```python
from build123d import *

# Parameters (mm, degrees)
F0_R     = 11.0625
F1_DEPTH = 11
F2_R     = 5
F3_SIZE  = 2
F4_SIZE  = 2


# Not quite as in the source:
# - a feature names something its author has since deleted; it is built from what else it names


with BuildPart() as f1:
    # F0 (on Top) → F1 (new body)
    with BuildSketch(Plane.XY):
        Polygon((12.7279220614, 42.7279220614), (0, 48), (-12.7279220614, 42.7279220614), (-18, 30), (-12.7279220614, 17.2720779386), (-21.3220193017, 2.3866648732), (-34.9807621135, 0.5884572681), (-43.3674269867, -10.3412571882), (-41.5692193817, -24), (-30.6395049254, -32.3866648732), (-16.9807621135, -30.5884572681), (-8.5940972403, -19.6587428118), (8.5940972403, -19.6587428118), (16.9807621135, -30.5884572681), (30.6395049254, -32.3866648732), (41.5692193817, -24), (43.3674269867, -10.3412571882), (34.9807621135, 0.5884572681), (21.3220193017, 2.3866648732), (12.7279220614, 17.2720779386), (18, 30), align=None)
        with Locations((-25.9807621135, -15)):
            Circle(F0_R, mode=Mode.SUBTRACT)
        Circle(F0_R, mode=Mode.SUBTRACT)
        with Locations((25.9807621135, -15)):
            Circle(F0_R, mode=Mode.SUBTRACT)
        with Locations((0, 30)):
            Circle(F0_R, mode=Mode.SUBTRACT)
    extrude(amount=F1_DEPTH)

    # F2
    f2_edges = [f1.edges().sort_by_distance(p)[0] for p in [
        (-16.980762, -30.588457, 5.5),
        (-30.639505, -32.386665, 5.5),
        (-41.569219, -24, 5.5),
        (-43.367427, -10.341257, 5.5),
        (-34.980762, 0.588457, 5.5),
        (-18, 30, 5.5),
        (-12.727922, 42.727922, 5.5),
        (0, 48, 5.5),
        (12.727922, 42.727922, 5.5),
        (34.980762, 0.588457, 5.5),
        (43.367427, -10.341257, 5.5),
        (41.569219, -24, 5.5),
        (30.639505, -32.386665, 5.5),
        (16.980762, -30.588457, 5.5),
        (8.594097, -19.658743, 5.5),
        (-8.594097, -19.658743, 5.5),
        (18, 30, 5.5),
        (-12.727922, 17.272078, 5.5),
        (-21.322019, 2.386665, 5.5),
    ]]
    fillet(f2_edges, radius=F2_R)

    # F3
    f3_edges = [f1.edges().sort_by_distance(p)[0] for p in [
        (27.124716, 1.622725, 11),
        (34.774782, 0.231689, 11),
        (17.024971, 9.829371, 11),
        (39.174095, -4.8764, 11),
        (14.967679, 22.67933, 11),
        (42.969503, -10.447881, 11),
        (17.588039, 30, 11),
        (42.468323, -17.170629, 11),
        (15.363961, 36.363961, 11),
        (41.212451, -23.794019, 11),
        (12.436622, 42.436622, 11),
        (36.104362, -28.193332, 11),
        (6.363961, 45.363961, 11),
        (30.532882, -31.988741, 11),
        (0, 47.588039, 11),
        (23.810134, -31.487561, 11),
        (-6.363961, 45.363961, 11),
        (17.186743, -30.231689, 11),
        (-12.436622, 42.436622, 11),
        (12.907556, -25.280152, 11),
        (-15.363961, 36.363961, 11),
        (8.339814, -20.174379, 11),
        (-17.588039, 30, 11),
        (0, -19.658743, 11),
        (-15.439476, 23.818348, 11),
        (-8.339814, -20.174379, 11),
        (-13.301618, 17.30968, 11),
        (-12.907556, -25.280152, 11),
        (-17.024971, 9.829371, 11),
        (-17.186743, -30.231689, 11),
        (-21.641432, 2.864699, 11),
        (-23.810134, -31.487561, 11),
        (-28.347032, 1.461804, 11),
        (-30.532882, -31.988741, 11),
        (-34.774782, 0.231689, 11),
        (-36.104362, -28.193332, 11),
        (-39.174095, -4.8764, 11),
        (-41.212451, -23.794019, 11),
        (-42.969503, -10.447881, 11),
        (-42.468323, -17.170629, 11),
        (-37.043262, -15, 11),
        (-11.0625, 0, 11),
        (14.918262, -15, 11),
        (-11.0625, 30, 11),
    ]]
    chamfer(f3_edges, length=F3_SIZE)

    # F4
    f4_edges = [f1.edges().sort_by_distance(p)[0] for p in [
        (27.124716, 1.622725, 0),
        (34.774782, 0.231689, 0),
        (17.024971, 9.829371, 0),
        (39.174095, -4.8764, 0),
        (14.967679, 22.67933, 0),
        (42.969503, -10.447881, 0),
        (17.588039, 30, 0),
        (42.468323, -17.170629, 0),
        (15.363961, 36.363961, 0),
        (41.212451, -23.794019, 0),
        (12.436622, 42.436622, 0),
        (36.104362, -28.193332, 0),
        (6.363961, 45.363961, 0),
        (30.532882, -31.988741, 0),
        (0, 47.588039, 0),
        (23.810134, -31.487561, 0),
        (-6.363961, 45.363961, 0),
        (17.186743, -30.231689, 0),
        (-12.436622, 42.436622, 0),
        (12.907556, -25.280152, 0),
        (-15.363961, 36.363961, 0),
        (8.339814, -20.174379, 0),
        (-17.588039, 30, 0),
        (0, -19.658743, 0),
        (-15.439476, 23.818348, 0),
        (-8.339814, -20.174379, 0),
        (-13.301618, 17.30968, 0),
        (-12.907556, -25.280152, 0),
        (-17.024971, 9.829371, 0),
        (-17.186743, -30.231689, 0),
        (-21.641432, 2.864699, 0),
        (-23.810134, -31.487561, 0),
        (-28.347032, 1.461804, 0),
        (-30.532882, -31.988741, 0),
        (-34.774782, 0.231689, 0),
        (-36.104362, -28.193332, 0),
        (-39.174095, -4.8764, 0),
        (-41.212451, -23.794019, 0),
        (-42.969503, -10.447881, 0),
        (-42.468323, -17.170629, 0),
        (-37.043262, -15, 0),
        (-11.0625, 0, 0),
        (14.918262, -15, 0),
        (-11.0625, 30, 0),
    ]]
    chamfer(f4_edges, length=F4_SIZE)


solid = f1.part
```
Verification items for the finished model (mm, model axes). A direction names the side the tool comes from. Round coordinates to 2 decimals unless told otherwise and drop trailing zeros. Order: outer loops, then holes, each group sorted by start corner. A loop starts at its lowest first (then second) coordinate and runs counter-clockwise, first axis right, second up. Notation, with made-up numbers: (82.25, 4.5) - (129.25, 4.5) arc R31 cw to (129.25, 38.5) - close; hole circle Ø6 at (10.25, -31). An arc over 180 degrees is marked (long way). Use CSV: the item, a comma, the result in double quotes.
(1) Thickness scan on probe 1 along Y at (x, z) = (0, 6.5); probe 2 along Y at (x, z) = (4, 3.5); probe 3 along X at (y, z) = (-25, 1.5). Record the ranges inside material, lowest first. Write a range as from..to.
Entries:
probe 1,"-19.66..-11.06, 11.06..18.94, 41.06..47.59"
probe 2,"-19.66..-10.31, 10.31..19.69, 40.31..46.34"
probe 3,"-39.44..-31.79, -20.18..-13.32, 13.32..20.18, 31.79..39.44"
(2) Access from +Z, -Z, +X, -X, +Y, -Y to the whole of each face (thin tool, end or side, straight path). Record for faces 1 (the face through (-24.006, -30.519, 1.014)), 2 (the face through (8.37, -20.19, 5.55)), 3 (the face through (13.65, -24.629, 9.986)), 4 (the face through (16.238, 9.22, 9.986)).
Entries:
face 1,"-Z, -Y"
face 2,"+Z, -Z, -Y"
face 3,"+Z, -Y"
face 4,"+Z, +X"
(3) Section check A-A on x = 0. Record the boundary of the cut face in (y, z).
Entries:
outline,"(-19.66, 2) - (-17.66, 0) - (-13.06, 0) - (-11.06, 2) - (-11.06, 9) - (-13.06, 11) - (-17.66, 11) - (-19.66, 9) - close; (11.06, 2) - (13.06, 0) - (16.94, 0) - (18.94, 2) - (18.94, 9) - (16.94, 11) - (13.06, 11) - (11.06, 9) - close; (41.06, 2) - (43.06, 0) - (45.59, 0) - (47.59, 2) - (47.59, 9) - (45.59, 11) - (43.06, 11) - (41.06, 9) - close"
(4) Section check C-C on y = -15. Record the boundary of the cut face in (x, z).
Entries:
outline,"(-42.75, 2) - (-40.74, 0) - (-39.04, 0) - (-37.04, 2) - (-37.04, 9) - (-39.04, 11) - (-40.74, 11) - (-42.75, 9) - close; (-14.92, 2) - (-12.92, 0) - (12.92, 0) - (14.92, 2) - (14.92, 9) - (12.92, 11) - (-12.92, 11) - (-14.92, 9) - close; (37.04, 2) - (39.04, 0) - (40.74, 0) - (42.75, 2) - (42.75, 9) - (40.74, 11) - (39.04, 11) - (37.04, 9) - close"
(5) Gauge pin test, flat ends, axial feed: pin 1 Ø2 at (y, z) = (-23, 8) entering from -X; pin 2 Ø13.5 at (x, y) = (-25.98, -15) entering from -Z; pin 3 Ø3 at (y, z) = (14, 3) entering from -X. Record the tip position at first contact, or that the pin passes through.
Entries:
pin 1,"x = -41.83"
pin 2,"through"
pin 3,"x = -15.48"
(6) Section check D-D on z = 5. State how many separate pieces and enclosed holes the cut face has, and give its area (3 significant figures).
Entries:
separate pieces,"1"
enclosed holes,"4"
area,"2,170 mm^2"
(7) Section check B-B on y = 30. Record the boundary of the cut face in (x, z).
Entries:
outline,"(-17.59, 2) - (-15.59, 0) - (-13.06, 0) - (-11.06, 2) - (-11.06, 9) - (-13.06, 11) - (-15.59, 11) - (-17.59, 9) - close; (11.06, 2) - (13.06, 0) - (15.59, 0) - (17.59, 2) - (17.59, 9) - (15.59, 11) - (13.06, 11) - (11.06, 9) - close"
